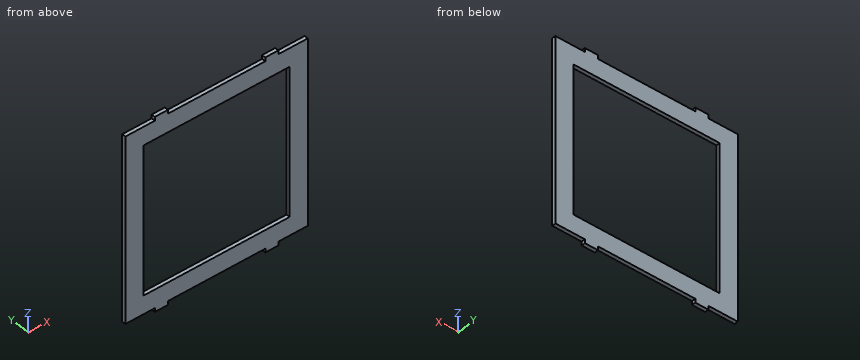
from build123d import *

# Parameters (mm, degrees)
F0_W     = 79.375
F0_H     = 79.375
F1_DEPTH = 2.032


with BuildPart() as f1:
    # F0 (on Front) → F1 (new body)
    with BuildSketch(Plane.XZ):
        Polygon((-33.528, 49.53), (-49.53, 49.53), (-49.53, 0), (-49.53, -49.53), (-33.528, -49.53), (-33.528, -51.562), (-26.416, -51.562), (-26.416, -49.53), (26.416, -49.53), (26.416, -51.562), (33.528, -51.562), (33.528, -49.53), (49.53, -49.53), (49.53, 0), (49.53, 49.53), (33.528, 49.53), (33.528, 51.562), (26.416, 51.562), (26.416, 49.53), (-26.416, 49.53), (-26.416, 51.562), (-33.528, 51.562), align=None)
        Rectangle(F0_W, F0_H, mode=Mode.SUBTRACT)
    extrude(amount=F1_DEPTH)


solid = f1.part
The model under review builds one solid part; all positions refer to its coordinate system, in mm. Give positions to 0.01 mm unless a question says otherwise; leave off trailing zeros. Order: outer loops, then holes, each group sorted by start corner. A loop starts at its lowest first (then second) coordinate and runs counter-clockwise, first axis right, second up. Notation, with made-up numbers: M 29.5,-27.75 L 69.5,-27.75 A26 cw 69.5,-5.75 Z; hole C 89.5,43 d2. An arc over 180 degrees is marked long. Answer in a Markdown table with one row per item. Add a question column.
1. Add section C-C on y = -0.8. State the section outline as (x, z) points, plus the area to 3 significant figures.
2. For pin 1 Ø1 at (x, y) = (-10.5, -1) entering from +Z; pin 2 Ø0.6 at (x, y) = (1, -1.5) entering from -Z; pin 3 Ø0.6 at (y, z) = (-1.5, -51) entering from -X, all flat-tipped, find the tip position at first contact; note any pin that passes through.
3. Add section A-A on z = 0.5. State the section outline as (x, y) points.
4. To check wall thickness, follow line 1 along X through (y, z) = (-1.25, -17); line 2 along Z through (x, y) = (-27, -0.15). State the ranges of each line that lie inside material, in increasing order.
5. Add section B-B on x = 10. State the section outline as (y, z) points, plus the area to 3 significant figures.
The answers:
| question | item | result |
|---|---|---|
| 1 | outline | M -49.53,-49.53 L -33.53,-49.53 L -33.53,-51.56 L -26.42,-51.56 L -26.42,-49.53 L 26.42,-49.53 L 26.42,-51.56 L 33.53,-51.56 L 33.53,-49.53 L 49.53,-49.53 L 49.53,49.53 L 33.53,49.53 L 33.53,51.56 L 26.42,51.56 L 26.42,49.53 L -26.42,49.53 L -26.42,51.56 L -33.53,51.56 L -33.53,49.53 L -49.53,49.53 Z; hole M -39.69,-39.69 L 39.69,-39.69 L 39.69,39.69 L -39.69,39.69 Z |
| 1 | area | 3,570 mm2 |
| 2 | pin 1 | z = 49.53 |
| 2 | pin 2 | z = -49.53 |
| 2 | pin 3 | x = -33.53 |
| 3 | outline | M -49.53,-2.03 L -39.69,-2.03 L -39.69,0 L -49.53,0 Z; M 39.69,-2.03 L 49.53,-2.03 L 49.53,0 L 39.69,0 Z |
| 4 | line 1 | -49.53 to -39.69, 39.69 to 49.53 |
| 4 | line 2 | -51.56 to -39.69, 39.69 to 51.56 |
| 5 | outline | M -2.03,-49.53 L 0,-49.53 L 0,-39.69 L -2.03,-39.69 Z; M -2.03,39.69 L 0,39.69 L 0,49.53 L -2.03,49.53 Z |
| 5 | area | 40.0 mm2 |
